Work out the finished part from the listing and answer in its coordinate system (mm). Face numbers are marked on the shaded views. A direction names the side the tool comes from. Coordinates: 2 decimals unless noted, no trailing zeros. Loops run counter-clockwise (first coordinate to the right, second up) from the corner with the lowest first, then second, coordinate; pieces in that order, holes last. Notation, with made-up numbers: (-13, 40) -> (11, 40) arc R25 ccw to (11, 75) -> close; hole circle Ø5 at (21.5, -28). An arc over 180 degrees is marked (long way). Use a Markdown table: item, result. Add a question column.
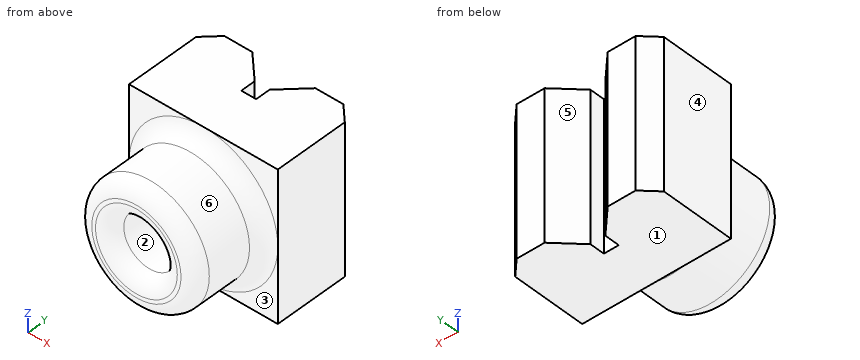
```python
from build123d import *

# Parameters (mm, degrees)
F1_DEPTH = 10
F2_R     = 4
F2_R_2   = 1.75
F3_DEPTH = 5
F4_SIZE  = 1
F5_W     = 1
F5_H     = 2.3880545414
F6_DEPTH = 25
F7_R     = 0.99999


# Not quite as in the source:
# - a fillet or chamfer is up to 0.001 mm smaller than in the source, because OpenCascade refuses the exact size


with BuildPart() as f1:
    # F0 (on Top) → F1 (new body)
    with BuildSketch(Plane.XY):
        Polygon((0, 6), (0, 0), (10, 0), (10, 6), (7.1213203436, 6), (5, 3.8786796564), (2.8786796564, 6), align=None)
    extrude(amount=F1_DEPTH)

    # F2 (on face) → F3 (join)
    with BuildSketch(Plane.XZ):
        with Locations((5, 5)):
            Circle(F2_R)
        with Locations((5, 5)):
            Circle(F2_R_2, mode=Mode.SUBTRACT)
    extrude(amount=F3_DEPTH)

    # F4
    f4_edges = [f1.edges().sort_by_distance(p)[0] for p in [
        (10, 6, 5),
        (0, 6, 5),
    ]]
    chamfer(f4_edges, length=F4_SIZE)

    # F5 (on face) → F6 (cut)
    with BuildSketch(Plane(origin=(0, 0, 0), x_dir=(1, 0, 0), z_dir=(0, 0, -1))):
        with Locations((5, -4.5727069271)):
            Rectangle(F5_W, F5_H)
    extrude(amount=-F6_DEPTH, mode=Mode.SUBTRACT)

    # F7 (radius 1 in the source; OpenCascade refuses exactly that, so slightly less here)
    f7_edges = [f1.edges().sort_by_distance(p)[0] for p in [
        (1, 0, 5),
        (1, -5, 5),
        (3.25, -5, 5),
    ]]
    fillet(f7_edges, radius=F7_R)


solid = f1.part
```
Item 1: For a pull along Z with two mould halves and no side action, classify the marked faces 1, 2 and 3 as +Z half, -Z half, draft (parallel to the pull), parting line (faces both ways), or undercut.
Item 2: Find the intervals of material crossed by probe 1 along Z at (x, y) = (5, -1.1); probe 2 along X at (y, z) = (-3.5, 4.75); probe 3 along X at (y, z) = (4.5, 1), in increasing order.
Item 3: Given pin 1 (1.1 mm diameter, centred on x = 5, z = 5.5, fed in from +Y); pin 2 (1 mm diameter, centred on x = 5, z = 4.5, fed in from -Y); pin 3 (2 mm diameter, centred on x = 3, y = -1.5, fed in from +Z), each flat-ended and moving along its own axis, determine where each tip first touches the part or whether it passes through.
Item 4: For the marked faces 4, 5 and 6, determine the directions among +Z, -Z, +X, -X, +Y, -Y from which every point of the face is accessible in a straight line to the end or side of a thin tool.
Item 5: Section C-C (y = -2.25) is taken. Determine the outline of the cut face in (x, z).
Output:
| question | item | result |
|---|---|---|
| 1 | face 1 | -Z half |
| 1 | face 2 | undercut |
| 1 | face 3 | draft |
| 2 | probe 1 | z = 1 to 3.25, 6.75 to 9 |
| 2 | probe 2 | x = 1.01 to 3.27, 6.73 to 8.99 |
| 2 | probe 3 | x = 0 to 4.38, 5.62 to 10 |
| 3 | pin 1 | stops at y = 4.43 |
| 3 | pin 2 | stops at y = 0 |
| 3 | pin 3 | stops at z = 8.87 |
| 4 | face 4 | +Z, -Z, -X, +Y, -Y |
| 4 | face 5 | +Z, -Z, +Y |
| 4 | face 6 | -Y |
| 5 | outline | circle Ø8 at (5, 5); hole circle Ø3.5 at (5, 5) |
